Read the model definition and answer for the solid it produces. Units are mm, in the model's axes. A direction names the side the tool comes from. Coordinates: 2 decimals unless noted, no trailing zeros. Write each loop counter-clockwise with the first axis right and the second up, starting at its lowest first coordinate (ties: lowest second). Pieces come first, ordered by that corner, then holes. Notation, with made-up numbers: (31.25, 31) -> (78.25, 31) arc R21 cw to (78.25, 54) -> close; hole circle Ø7 at (68, 67.5). An arc over 180 degrees is marked (long way). Write item = value, one per line. Start each with the question number.
1) For a pull along X with two mould halves and no side action, classify faces 4 (the face through (-5.458, 6.002, 18.241)), 5 (the face through (6.864, -0.49, 18.241)), 6 (the face through (-6.72, -1.46, 18.24)) as released by +X, released by -X, zero draft, split by the parting line, or undercut.
2) Flat-ended cylindrical pins translate along their axes: pin 1 Ø10 at (y, z) = (6.5, 30) entering from -X; pin 2 Ø1 at (y, z) = (-7, 20) entering from +X; pin 3 Ø1 at (y, z) = (-1, 8.5) entering from -X. Find the tip coordinate at first contact, or state that the pin passes through.
3) Section B-B (y = -2.5) is taken. Determine the outline of the cut face in (x, z), plus the area to 3 significant figures.
4) Section A-A (y = -5) is taken. Determine the outline of the cut face in (x, z), plus the area to 3 significant figures.
5) A tool of negligible diameter and unlimited length cuts with its end or side. For faces 1 (the face through (5.477, 6.014, 18.241)), 2 (the face through (-5.164, -6.257, 18.241)), 3 (the face through (5.173, -6.277, 18.241)), from which of +Z, -Z, +X, -X, +Y, -Y can it reach the whole face along a straight path? Write none if from no direction.
6) Find the intervals of material crossed by line 1 along Y through (x, z) = (-7, 17.5); line 2 along X through (y, z) = (-6.25, 24); line 3 along X through (y, z) = (7.5, 21.5), in increasing order. Write a range as from..to.
from build123d import *

# Parameters (mm, degrees)
SKETCH1_R               = 9.7778
BOSS_EXTRUDE1_DEPTH     = 37
CUT_EXTRUDE1_DEPTH      = 40.499503107
CUT_EXTRUDE2_DEPTH      = 40.499503107
CUT_EXTRUDE2_DEPTH_BACK = 40.499503107
SKETCH4_R               = 5.75
CIRPATTERN1_COUNT       = 11


with BuildPart() as part:
    # Sketch1 → Boss-Extrude1 (new body)
    with BuildSketch(Plane.XY):
        Circle(SKETCH1_R)
    extrude(amount=BOSS_EXTRUDE1_DEPTH)

    # Sketch2 → Cut-Extrude1 (cut, through all)
    with BuildSketch(Plane.XY):
        Polygon((0, 6.440231992), (-0.998470792, 7.29965938), (-1.704297747, 8.720724317), (-2.306603416, 9.501839481), (-1.704297747, 10.285038999), (0, 10.999278518), (1.704297747, 10.285038999), (2.306603416, 9.501839481), (1.704297747, 8.720724317), (0.998470792, 7.29965938), align=None)
    cut_extrude1 = extrude(amount=CUT_EXTRUDE1_DEPTH, mode=Mode.SUBTRACT)

    # Sketch4 → Cut-Extrude2 (cut, two sides: drawn at the far end of the back side and taken through both)
    with BuildSketch(Plane.XY.offset(37).offset(-CUT_EXTRUDE2_DEPTH_BACK)):
        Circle(SKETCH4_R)
    extrude(amount=CUT_EXTRUDE2_DEPTH + CUT_EXTRUDE2_DEPTH_BACK, mode=Mode.SUBTRACT)

    # CirPattern1: Cut-Extrude1 ×11 about axis
    cirpattern1_axis = Axis((0, 0, 0), (0, 0, 1))
    for i in range(1, CIRPATTERN1_COUNT):
        add(cut_extrude1.rotate(cirpattern1_axis, i * 360 / CIRPATTERN1_COUNT), mode=Mode.SUBTRACT)


solid = part.part
Answer key:
q1.face_4 = undercut
q1.face_5 = released by +X
q1.face_6 = released by -X
q2.pin_1 = -9.66
q2.pin_2 = 5.58
q2.pin_3 = -6.85
q3.outline = (-7.77, 0) -> (-5.18, 0) -> (-5.18, 37) -> (-7.77, 37) -> close; (5.18, 0) -> (7.77, 0) -> (7.77, 37) -> (5.18, 37) -> close
q3.area = 192 mm^2
q4.outline = (-4.86, 0) -> (-2.84, 0) -> (-2.84, 37) -> (-4.86, 37) -> close; (2.84, 0) -> (4.86, 0) -> (4.86, 37) -> (2.84, 37) -> close
q4.area = 150 mm^2
q5.face_1 = +Z, -Z, +Y
q5.face_2 = +Z, -Z, -X
q5.face_3 = +Z, -Z, +X
q6.line_1 = -4.24..-1.9, -0.37..2.15, 4.9..6.72
q6.line_2 = -5.16..-1.97, -1.77..1.77, 1.97..5.16
q6.line_3 = -3.2..-1.1, 1.1..3.2
